Geometry: final body of the model. Coordinates: model frame, mm. A direction names the side the tool comes from. Give positions to 0.01 mm unless a question says otherwise; leave off trailing zeros. Order: outer loops, then holes, each group sorted by start corner. A loop starts at its lowest first (then second) coordinate and runs counter-clockwise, first axis right, second up. Notation, with made-up numbers: M 49.25,38.5 L 65.25,38.5 A28 ccw 65.25,60.5 Z; hole C -36.5,60 d5. An arc over 180 degrees is marked long. Use CSV: the item, a comma, the result in double quotes.
```python
from build123d import *

# Parameters (mm, degrees)
SKETCH1_W           = 25.4
SKETCH1_H           = 60.96
BOSS_EXTRUDE1_DEPTH = 19.05
SKETCH3_W           = 17.78
SKETCH3_H           = 14.732
CUT_EXTRUDE1_DEPTH  = 19.05
SKETCH5_R           = 3.175
CUT_EXTRUDE3_DEPTH  = 58.42


with BuildPart() as part:
    # Sketch1 → Boss-Extrude1 (new body)
    with BuildSketch(Plane(origin=(0, 0, 0), x_dir=(1, 0, 0), z_dir=(0, 1, 0))):
        with Locations((12.7, 30.48)):
            Rectangle(SKETCH1_W, SKETCH1_H)
    extrude(amount=BOSS_EXTRUDE1_DEPTH)

    # Sketch3 → Cut-Extrude1 (cut)
    with BuildSketch(Plane(origin=(0, 19.05, 0), x_dir=(1, 0, 0), z_dir=(0, 1, 0))):
        with Locations((12.7, 30.48)):
            Rectangle(SKETCH3_W, SKETCH3_H)
    extrude(amount=-CUT_EXTRUDE1_DEPTH, mode=Mode.SUBTRACT)

    # Sketch5 → Cut-Extrude3 (cut)
    with BuildSketch(Plane.XY):
        with Locations((12.7, 13.6525)):
            Circle(SKETCH5_R)
    extrude(amount=-CUT_EXTRUDE3_DEPTH, mode=Mode.SUBTRACT)


solid = part.part
```
1. Line query: line 1 (X direction, y = 9.5, z = -28); line 2 (Z direction, x = 8.25, y = 6.5); line 3 (Y direction, x = 12.7, z = -10.75). Output: solid intervals per line, ascending.
Answer:
line 1,"0 to 3.81, 21.59 to 25.4"
line 2,"-60.96 to -37.85, -23.11 to 0"
line 3,"0 to 10.48, 16.83 to 19.05"
2. Section C-C, the plane y = 4.5. Return the cut outline in (x, z), plus the area to 3 significant figures.
Answer:
outline,"M 0,-60.96 L 25.4,-60.96 L 25.4,0 L 0,0 Z; hole M 3.81,-37.85 L 21.59,-37.85 L 21.59,-23.11 L 3.81,-23.11 Z"
area,"1,290 mm2"
3. Pin query (flat end, axial travel): pin 1 Ø6 at (x, y) = (7.5, 14.5) entering from +Z; pin 2 Ø2 at (x, z) = (18.5, -25) entering from +Y; pin 3 Ø5 at (x, y) = (12.7, 13.65) entering from +Z. Return the tip coordinate at first contact, or that it passes through.
Answer:
pin 1,"z = 0"
pin 2,"through"
pin 3,"z = -58.42"
4. Section D-D, the plane x = 12.7. Return the cut outline in (y, z).
Answer:
outline,"M 0,-60.96 L 19.05,-60.96 L 19.05,-37.85 L 16.83,-37.85 L 16.83,-58.42 L 10.48,-58.42 L 10.48,-37.85 L 0,-37.85 Z; M 0,-23.11 L 10.48,-23.11 L 10.48,0 L 0,0 Z; M 16.83,-23.11 L 19.05,-23.11 L 19.05,0 L 16.83,0 Z"
5. Section B-B, the plane z = -37. Return the cut outline in (x, y), plus the area to 3 significant figures.
Answer:
outline,"M 0,0 L 3.81,0 L 3.81,19.05 L 0,19.05 Z; M 21.59,0 L 25.4,0 L 25.4,19.05 L 21.59,19.05 Z"
area,"145 mm2"
6. Pull-direction query (Z, two-part tool) for faces 4 (the face through (13, 9, -60.96)), 5 (the face through (21.59, 10, -30)), 6 (the face through (13, 10, -37.846)), 7 (the face through (10.18, 11.72, -47.99)); classes: +Z half, -Z half, draft (parallel to the pull), parting line (faces both ways), or undercut.
Answer:
face 4,"-Z half"
face 5,"undercut"
face 6,"undercut"
face 7,"draft"
7. Section A-A, the plane x = 17.25. Return the cut outline in (y, z), plus the area to 3 significant figures.
Answer:
outline,"M 0,-60.96 L 19.05,-60.96 L 19.05,-37.85 L 0,-37.85 Z; M 0,-23.11 L 19.05,-23.11 L 19.05,0 L 0,0 Z"
area,"881 mm2"
8. Reachability of faces 1 (the face through (3.81, 10, -30)), 2 (the face through (13, 9, 0)), 3 (the face through (10.18, 11.72, -11.4)) from +Z, -Z, +X, -X, +Y, -Y: full face, straight path, thin tool, end or side. Return the list, or none.
Answer:
face 1,"+Y, -Y"
face 2,"+Z, +X, -X, +Y, -Y"
face 3,"+Z"
